Geometry check sheet. Reference: drawing and pictorial views, mm from the part's lowest x, y, z. Round coordinates to 2 decimals unless told otherwise and drop trailing zeros. Order: outer loops, then holes, each group sorted by start corner. A loop starts at its lowest first (then second) coordinate and runs counter-clockwise, first axis right, second up. Notation, with made-up numbers: (12.5, 60.5) -> (30.5, 60.5) arc R18 cw to (30.5, 70.5) -> close; hole circle Ø1 at (-28, -25.75). An arc over 180 degrees is marked (long way). Return JSON: item names as keys, results as strings. Group by question number.
1) Scan lines: L1, parallel to Z at x = 40, y = 4 (1 decimal); L2, parallel to X at y = 4.5, z = 6 (1 decimal); L3, parallel to X at y = 9.5, z = 13 (1 decimal). Record each from-to range of solid material in increasing order.
2) Section check A-A on x = 40. Enter the section's corners in (y, z) (1 decimal), plus the area to 3 significant figures.
3) Section check C-C on z = 12.5. Enter the section's corners in (x, y) (1 decimal), plus the area to 3 significant figures.
4) Depth check by flat-ended pin: pin 1 (3 mm diameter, centred on y = 4.5, z = 12.5, fed in from -X). Enter the tip coordinate at first touch or a pass-through.
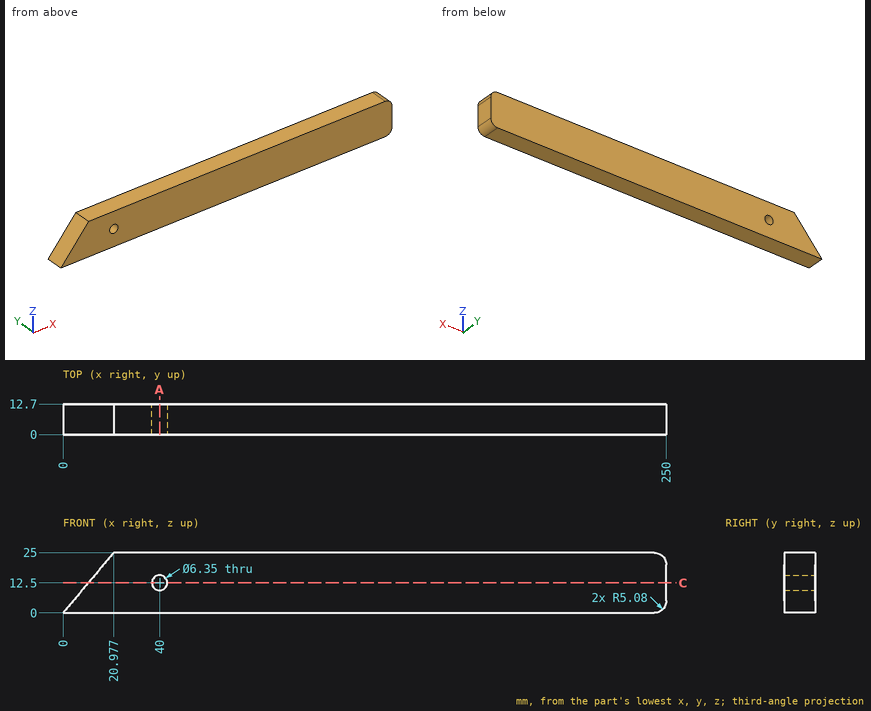
Check result:
{
 "1": {"L1": "0 to 9.3, 15.7 to 25", "L2": "5 to 250", "L3": "10.9 to 36.9, 43.1 to 250"},
 "2": {"outline": "(0, 0) -> (12.7, 0) -> (12.7, 9.3) -> (0, 9.3) -> close; (0, 15.7) -> (12.7, 15.7) -> (12.7, 25) -> (0, 25) -> close", "area": "237 mm^2"},
 "3": {"outline": "(10.5, 0) -> (36.8, 0) -> (36.8, 12.7) -> (10.5, 12.7) -> close; (43.2, 0) -> (250, 0) -> (250, 12.7) -> (43.2, 12.7) -> close", "area": "2,960 mm^2"},
 "4": {"pin 1": "x = 9.23"}
}
